Source: three-view drawing plus pictorial views. Frame: mm from the lowest corner of the part. Coordinates: 2 decimals unless noted, no trailing zeros. Loops run counter-clockwise (first coordinate to the right, second up) from the corner with the lowest first, then second, coordinate; pieces in that order, holes last.
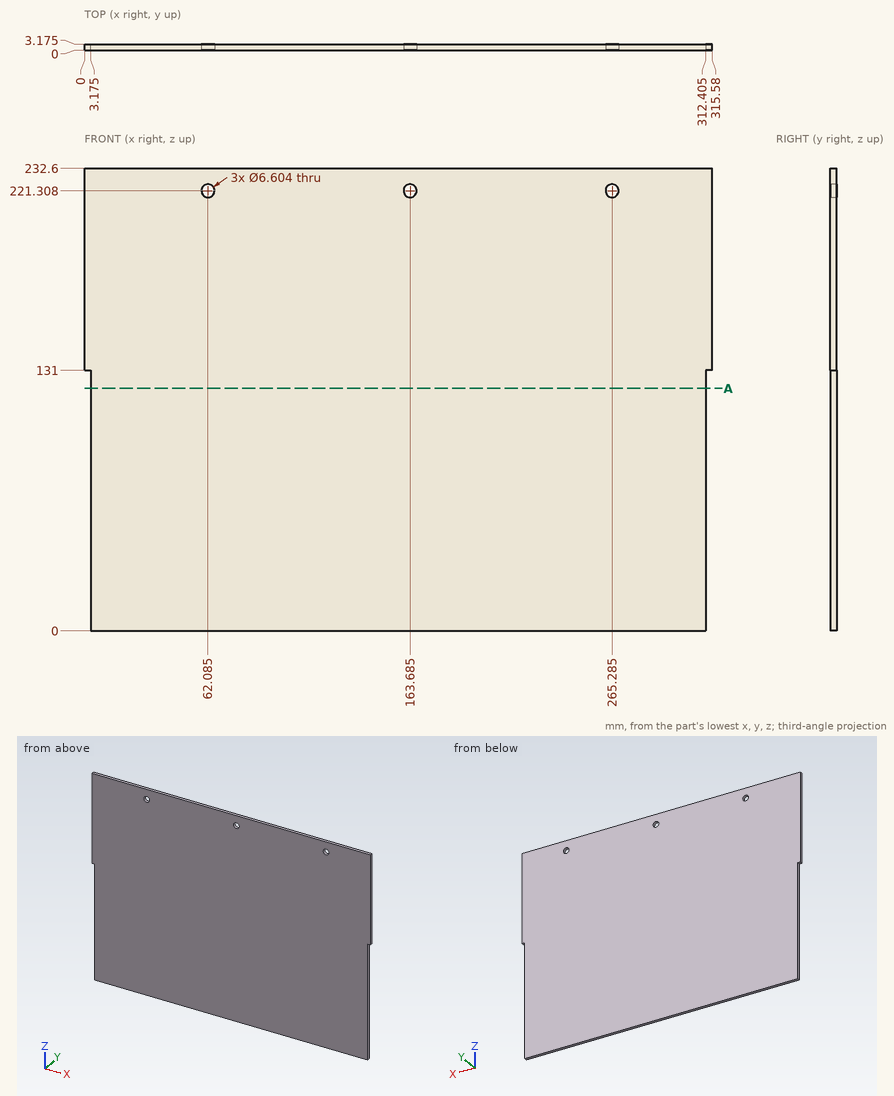
Q1. First-contact query: pin 1 Ø1 at (y, z) = (1, 73.5) entering from -X (3 decimals); pin 2 Ø1.6 at (x, y) = (1, 2.5) entering from -Z. Flat tips, straight axial feed; report the tip coordinate or a pass-through.
Q2. Material intervals for line 1 along X through (y, z) = (2.7, 20) (1 decimal); line 2 along Z through (x, y) = (266.5, 2.85), sorted ascending.
Q3. Section query A-A on z = 122. Return the cut outline in (x, y) (1 decimal).
Resolved:
1. pin 1: stops at x = 3.175
1. pin 2: stops at z = 131
2. line 1: x = 3.2 to 312.4
2. line 2: z = 0 to 218.24, 224.38 to 232.6
3. outline: (3.2, 0) - (312.4, 0) - (312.4, 3.2) - (3.2, 3.2) - close
